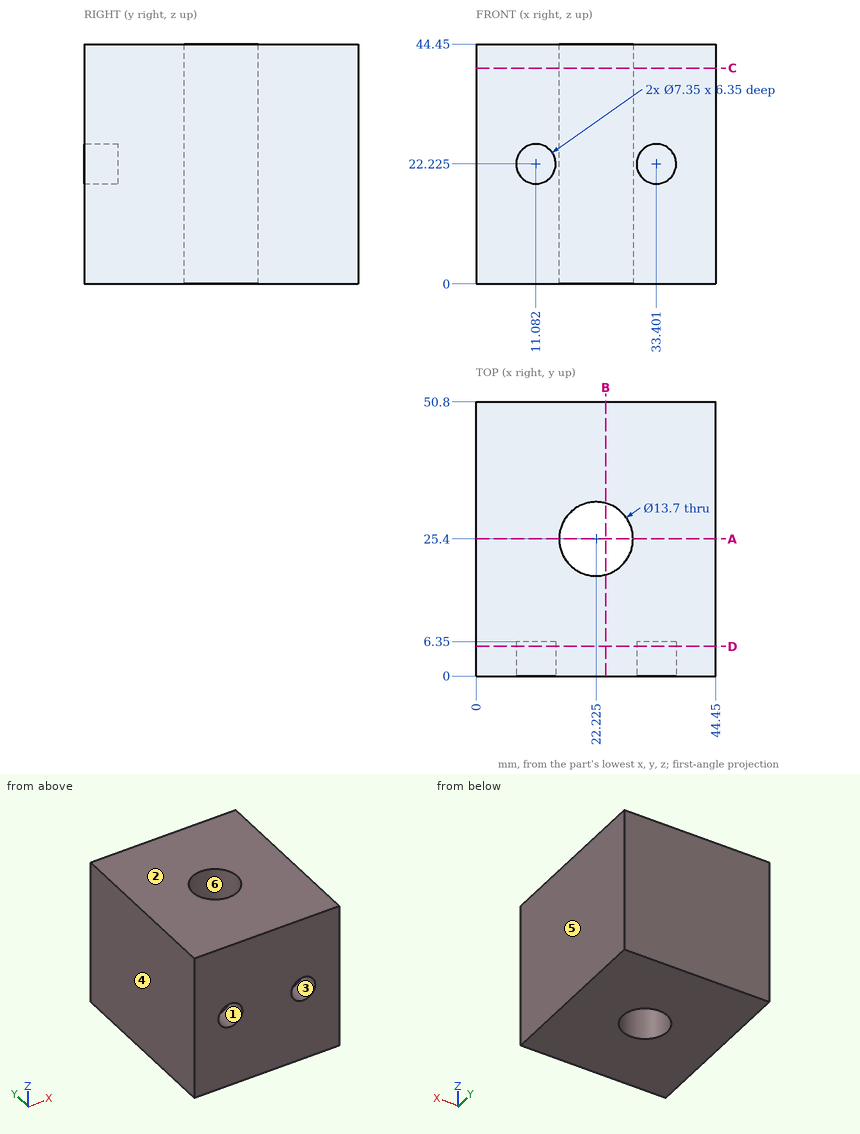
Answer from the drawing. Dimensions are ordinates in mm from the lowest x, y and z of the part. A direction names the side the tool comes from. Coordinates: 2 decimals unless noted, no trailing zeros. Write each loop counter-clockwise with the first axis right and the second up, starting at its lowest first coordinate (ties: lowest second). Pieces come first, ordered by that corner, then holes. Notation, with made-up numbers: M 59,59.5 L 88,59.5 A25 cw 88,95.5 Z; hole C 82,33 d5. An arc over 180 degrees is marked long. Put each result on its own line as item: value. Start each with the question number.
1. A cutting plane is placed at C-C on z = 40. Write down the section's boundary in (x, y) (3 decimals), then the cut area to 3 significant figures.
2. A cutting plane is placed at A-A on y = 25.4. Write down the section's boundary in (x, z) (3 decimals), then the cut area to 3 significant figures.
3. Which of the six approach directions +Z, -Z, +X, -X, +Y, -Y give full straight-line access (tool end or side, diameter ignored) to the marked faces 1 and 2?
4. A cutting plane is placed at B-B on x = 24. Write down the section's boundary in (y, z).
5. Flat-ended cylindrical pins translate along their axes: P1, Ø2, axis at x = 33.5, z = 21, coming from the -Y side; P2, Ø1, axis at x = 34.5, z = 33.5, coming from the -Y side; P3, Ø8, axis at x = 22.225, y = 25.4, coming from the -Z side. Find the tip coordinate at first contact, or state that the pin passes through.
6. A cutting plane is placed at D-D on y = 5.5. Write down the section's boundary in (x, z) (3 decimals).
7. For a pull along X with two mould halves and no side action, classify the marked faces 3, 4, 5 and 6 as pulls with the +X half, pulls with the -X half, needs draft (parallel to the pull), parting line crosses it, or undercut.
8. Consider line 1 (X direction, y = 25, z = 26); line 2 (X direction, y = 24, z = 18.5); line 3 (Y direction, x = 11, z = 25). Determine where each line is inside the solid, lowest interval first. Write a range as from..to.
Resolved:
1. outline: M 0,0 L 44.45,0 L 44.45,50.8 L 0,50.8 Z; hole C 22.225,25.4 d13.7
1. area: 2,110 mm2
2. outline: M 0,0 L 15.375,0 L 15.375,44.45 L 0,44.45 Z; M 29.075,0 L 44.45,0 L 44.45,44.45 L 29.075,44.45 Z
2. area: 1,370 mm2
3. face 1: -Y
3. face 2: +Z, +X, -X, +Y, -Y
4. outline: M 0,0 L 18.78,0 L 18.78,44.45 L 0,44.45 Z; M 32.02,0 L 50.8,0 L 50.8,44.45 L 32.02,44.45 Z
5. P1: stops at y = 6.35
5. P2: stops at y = 0
5. P3: passes through
6. outline: M 0,0 L 44.45,0 L 44.45,44.45 L 0,44.45 Z; hole C 11.082,22.225 d7.35; hole C 33.401,22.225 d7.35
7. face 3: undercut
7. face 4: pulls with the -X half
7. face 5: pulls with the +X half
7. face 6: undercut
8. line 1: x = 0..15.39, 29.06..44.45
8. line 2: x = 0..15.52, 28.93..44.45
8. line 3: y = 6.35..50.8
